Geometry check sheet. Reference: drawing and pictorial views, mm from the part's lowest x, y, z. A direction names the side the tool comes from. Give positions to 0.01 mm unless a question says otherwise; leave off trailing zeros. Order: outer loops, then holes, each group sorted by start corner. A loop starts at its lowest first (then second) coordinate and runs counter-clockwise, first axis right, second up. Notation, with made-up numbers: (15.25, -25) - (26.25, -25) arc R29 cw to (26.25, 4) - close; hole circle Ø11 at (62.5, -18). An arc over 180 degrees is marked (long way). Answer in a Markdown table with one row per item.
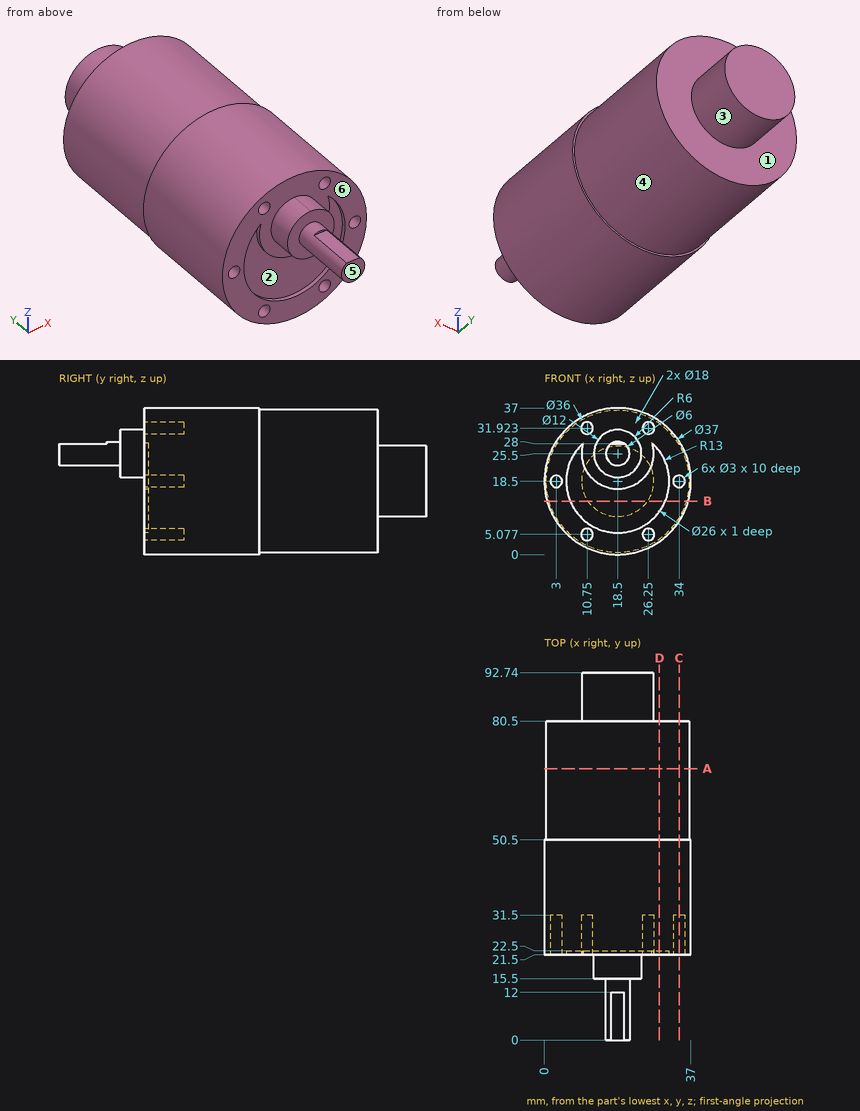
(1) Gauge pin test, flat ends, axial feed: P1, Ø2.5, axis at x = 18, y = 6.5, coming from the +Z side; P2, Ø2.5, axis at x = 26.25, z = 31.92, coming from the -Y side; P3, Ø2, axis at x = 29.5, z = 23.5, coming from the +Y side. Record the tip position at first contact, or that the pin passes through.
Geometry says:
| item | result |
|---|---|
| P1 | z = 28 |
| P2 | y = 31.5 |
| P3 | y = 80.5 |
(2) Cross-section at D-D, the plane x = 29. Record the cut outline in (y, z) (1 decimal).
Geometry says:
| item | result |
|---|---|
| outline | (21.5, 3.3) - (50.5, 3.3) - (50.5, 3.9) - (80.5, 3.9) - (80.5, 33.1) - (50.5, 33.1) - (50.5, 33.7) - (21.5, 33.7) - (21.5, 26.2) - (22.5, 26.2) - (22.5, 10.8) - (21.5, 10.8) - close |
(3) Cross-section at B-B, the plane z = 13.5. Record the cut outline in (x, y), then the cut area to 3 significant figures.
Geometry says:
| item | result |
|---|---|
| outline | (0.69, 21.5) - (6.5, 21.5) - (6.5, 22.5) - (30.5, 22.5) - (30.5, 21.5) - (36.31, 21.5) - (36.31, 50.5) - (35.79, 50.5) - (35.79, 80.5) - (25.98, 80.5) - (25.98, 92.74) - (11.02, 92.74) - (11.02, 80.5) - (1.21, 80.5) - (1.21, 50.5) - (0.69, 50.5) - close |
| area | 2,230 mm² |
(4) Cross-section at A-A, the plane y = 68.5. Record the cut outline in (x, z), then the cut area to 3 significant figures.
Geometry says:
| item | result |
|---|---|
| outline | circle Ø36 at (18.5, 18.5) |
| area | 1,020 mm² |
(5) Access from +Z, -Z, +X, -X, +Y, -Y to the whole of each face (thin tool, end or side, straight path). Record for the marked faces 4, 5 and 6.
Geometry says:
| item | result |
|---|---|
| face 4 | +Y |
| face 5 | +Z, -Z, +X, -X, -Y |
| face 6 | -Y |
(6) Thickness scan on L1, parallel to Z at x = 18, y = 22; L2, parallel to X at y = 22, z = 32; L3, parallel to X at y = 25, z = 18 (1 decimal). Record the ranges inside material, lowest first.
Geometry says:
| item | result |
|---|---|
| L1 | 0.01 to 5.51, 16.51 to 36.99 |
| L2 | 5.85 to 9.25, 12.25 to 24.75, 27.75 to 31.15 |
| L3 | 0 to 1.6, 4.4 to 32.6, 35.4 to 37 |
(7) Mould release check, pull along Z, two halves, no side actions. Record for the marked faces 1, 2 and 3: pulls with the +Z half, pulls with the -Z half, needs draft (parallel to the pull), parting line crosses it, or undercut.
Geometry says:
| item | result |
|---|---|
| face 1 | needs draft |
| face 2 | undercut |
| face 3 | parting line crosses it |
(8) Cross-section at C-C, the plane x = 34. Record the cut outline in (y, z), then the cut area to 4 significant figures.
Geometry says:
| item | result |
|---|---|
| outline | (21.5, 8.4) - (50.5, 8.4) - (50.5, 9.35) - (80.5, 9.35) - (80.5, 27.65) - (50.5, 27.65) - (50.5, 28.6) - (21.5, 28.6) - (21.5, 20) - (31.5, 20) - (31.5, 17) - (21.5, 17) - close |
| area | 1,105 mm² |
